```python
from build123d import *

# Parameters (mm, degrees)
SKETCH1_R           = 7.62
BOSS_EXTRUDE1_DEPTH = 12.7
CUT_EXTRUDE1_DEPTH  = 45.974


with BuildPart() as part:
    # Sketch1 → Boss-Extrude1 (new body)
    with BuildSketch(Plane(origin=(0, 0, 0), x_dir=(1, 0, 0), z_dir=(0, 1, 0))):
        with BuildLine():
            Line((0, 16.764), (254, 16.764))
            ThreePointArc((254, 16.764), (270.764, 0), (254, -16.764))
            Line((254, -16.764), (0, -16.764))
            ThreePointArc((0, -16.764), (-16.764, 0), (0, 16.764))
        make_face()
        with Locations(Location((0, 0, 0), (0, 0, 270))):
            Circle(SKETCH1_R, mode=Mode.SUBTRACT)
    extrude(amount=BOSS_EXTRUDE1_DEPTH)

    # Sketch3 → Cut-Extrude1 (cut)
    with BuildSketch(Plane(origin=(0, 12.7, 0), x_dir=(1, 0, 0), z_dir=(0, 1, 0))):
        with BuildLine():
            ThreePointArc((45.466, 7.62), (37.846, 0), (45.466, -7.62))
            Line((45.466, -7.62), (102.616, -7.62))
            Line((102.616, -7.62), (229.616, -7.62))
            ThreePointArc((229.616, -7.62), (237.236, 0), (229.616, 7.62))
            Line((229.616, 7.62), (167.898503034, 7.62))
            Line((167.898503034, 7.62), (45.466, 7.62))
        make_face()
    extrude(amount=-CUT_EXTRUDE1_DEPTH, mode=Mode.SUBTRACT)


solid = part.part
```
Geometry check sheet. Reference: the model listing, model coordinates, mm. A direction names the side the tool comes from. Coordinates: 2 decimals unless noted, no trailing zeros. Order: outer loops, then holes, each group sorted by start corner. A loop starts at its lowest first (then second) coordinate and runs counter-clockwise, first axis right, second up. Notation, with made-up numbers: (-13, 17.25) - (27, 17.25) arc R23 cw to (27, 45.25) - close; hole circle Ø7 at (-38, 74). An arc over 180 degrees is marked (long way). Use one line per item in the form item = value.
1. Access from +Z, -Z, +X, -X, +Y, -Y to the whole of each face (thin tool, end or side, straight path). Record for faces 4 (the face through (139, 6, -7.62)), 5 (the face through (270.76, 6.26, -0.37)).
Here are the results:
face_4 = +Y, -Y
face_5 = +X, +Y, -Y
2. Section check B-B (y = 6.5). Record the boundary of the cut face in (x, z).
Here are the results:
outline = (0, -16.76) - (254, -16.76) arc R16.76 ccw to (254, 16.76) - (0, 16.76) arc R16.76 ccw to start; hole circle Ø15.24 at (0, 0); hole (45.47, -7.62) - (229.62, -7.62) arc R7.62 ccw to (229.62, 7.62) - (45.47, 7.62) arc R7.62 ccw to start
3. Section check C-C (z = 0). Record the boundary of the cut face in (x, y), then the cut area to 3 significant figures.
Here are the results:
outline = (-16.76, 0) - (-7.62, 0) - (-7.62, 12.7) - (-16.76, 12.7) - close; (7.62, 0) - (37.85, 0) - (37.85, 12.7) - (7.62, 12.7) - close; (237.24, 0) - (270.76, 0) - (270.76, 12.7) - (237.24, 12.7) - close
area = 926 mm²
4. Gauge pin test, flat ends, axial feed: pin 1 (2 mm diameter, centred on y = 1.5, z = 11.5, fed in from +X); pin 2 (4 mm diameter, centred on y = 3, z = -11.5, fed in from +X); pin 3 (4 mm diameter, centred on y = 1.5, z = 5, fed in from +X); pin 4 (6 mm diameter, centred on x = 158.5, z = 4, fed in from -Y). Record the tip position at first contact, or that the pin passes through.
Here are the results:
pin_1 = 267.07
pin_2 = 267.81
pin_3 = 270.49
pin_4 = through
5. Section check A-A (x = 186). Record the boundary of the cut face in (y, z), then the cut area to 3 significant figures.
Here are the results:
outline = (0, -16.76) - (12.7, -16.76) - (12.7, -7.62) - (0, -7.62) - close; (0, 7.62) - (12.7, 7.62) - (12.7, 16.76) - (0, 16.76) - close
area = 232 mm²
6. Section check D-D (z = 11). Record the boundary of the cut face in (x, y), then the cut area to 3 significant figures.
Here are the results:
outline = (-12.65, 0) - (266.65, 0) - (266.65, 12.7) - (-12.65, 12.7) - close
area = 3,550 mm²
7. Scan lines: line 1 (X direction, y = 6.5, z = 0); line 2 (Z direction, x = 74.5, y = 9.5); line 3 (X direction, y = 7.5, z = 1). Record each from-to range of solid material in increasing order.
Here are the results:
line_1 = -16.76 to -7.62, 7.62 to 37.85, 237.24 to 270.76
line_2 = -16.76 to -7.62, 7.62 to 16.76
line_3 = -16.73 to -7.55, 7.55 to 37.91, 237.17 to 270.73
8. Draft check along Z on faces 1 (the face through (125, 6, -16.764)), 2 (the face through (136, 6, 7.62)), 3 (the face through (129, 6, 16.764)). Enter one of: pulls with the +Z half, pulls with the -Z half, needs draft (parallel to the pull), parting line crosses it, or undercut.
Here are the results:
face_1 = pulls with the -Z half
face_2 = undercut
face_3 = pulls with the +Z half
